from build123d import *

# Parameters (mm, degrees)
SKETCH1_W           = 59.0272
SKETCH1_H           = 30
BOSS_EXTRUDE1_DEPTH = 10
SKETCH2_R           = 2.1
CUT_EXTRUDE1_DEPTH  = 35.58399319
SKETCH3_R           = 1.7
CUT_EXTRUDE2_DEPTH  = 12
SKETCH4_R           = 1.65
CUT_EXTRUDE3_DEPTH  = 12
CUT_EXTRUDE4_DEPTH  = 2.5
CUT_EXTRUDE5_DEPTH  = 2.3
SKETCH7_R           = 3.5
CUT_EXTRUDE6_DEPTH  = 35.58399319
FILLET1_R           = 1
SKETCH8_W           = 39.5136
SKETCH8_H           = 30
CUT_EXTRUDE7_DEPTH  = 35.58399319


with BuildPart() as part:
    # Sketch1 → Boss-Extrude1 (new body)
    with BuildSketch(Plane(origin=(0, 0, 0), x_dir=(1, 0, 0), z_dir=(0, 1, 0))):
        Rectangle(SKETCH1_W, SKETCH1_H)
    extrude(amount=BOSS_EXTRUDE1_DEPTH)

    # Sketch2 → Cut-Extrude1 (cut, through all)
    with BuildSketch(Plane(origin=(0, 10, 0), x_dir=(1, 0, 0), z_dir=(0, 1, 0))):
        with Locations(Location((-6, -7.5, 0), (0, 0, 270))):
            Circle(SKETCH2_R)
        with Locations(Location((14, -7.5, 0), (0, 0, 270))):
            Circle(SKETCH2_R)
    extrude(amount=-CUT_EXTRUDE1_DEPTH, mode=Mode.SUBTRACT)

    # Sketch3 → Cut-Extrude2 (cut)
    with BuildSketch(Plane(origin=(29.5136, 0, 0), x_dir=(0, 0, -1), z_dir=(1, 0, 0))):
        with Locations((-10, 5)):
            Circle(SKETCH3_R)
        with Locations((10, 5)):
            Circle(SKETCH3_R)
    extrude(amount=-CUT_EXTRUDE2_DEPTH, mode=Mode.SUBTRACT)

    # Sketch4 → Cut-Extrude3 (cut)
    with BuildSketch(Plane.ZY.offset(29.5136)):
        with Locations((-10, 5)):
            Circle(SKETCH4_R)
        with Locations((10, 5)):
            Circle(SKETCH4_R)
    extrude(amount=-CUT_EXTRUDE3_DEPTH, mode=Mode.SUBTRACT)

    # Sketch5 → Cut-Extrude4 (cut)
    with BuildSketch(Plane(origin=(23.5136, 0, 0), x_dir=(0, 0, -1), z_dir=(1, 0, 0))):
        Polygon((-12.95, 6.703183294), (-12.95, 10), (-7.05, 10), (-7.05, 6.703183294), (-7.05, 3.296816706), (-10, 1.593633412), (-12.95, 3.296816706), align=None)
        Polygon((7.05, 6.703183294), (7.05, 3.296816706), (10, 1.593633412), (12.95, 3.296816706), (12.95, 6.703183294), (12.95, 10), (7.05, 10), align=None)
    extrude(amount=-CUT_EXTRUDE4_DEPTH, mode=Mode.SUBTRACT)

    # Sketch6 → Cut-Extrude5 (cut)
    with BuildSketch(Plane.ZY.offset(23.5136)):
        Polygon((-12.85, 6.645448267), (-12.85, 10), (-7.15, 10), (-7.15, 6.645448267), (-7.15, 3.354551733), (-10, 1.709103466), (-12.85, 3.354551733), align=None)
        Polygon((7.15, 6.645448267), (7.15, 3.354551733), (10, 1.709103466), (12.85, 3.354551733), (12.85, 6.645448267), (12.85, 10), (7.15, 10), align=None)
    extrude(amount=-CUT_EXTRUDE5_DEPTH, mode=Mode.SUBTRACT)

    # Sketch7 → Cut-Extrude6 (cut, through all)
    with BuildSketch(Plane(origin=(0, 10, 0), x_dir=(1, 0, 0), z_dir=(0, 1, 0))):
        with Locations(Location((9.7, 1.2, 0), (0, 0, 270))):
            Circle(SKETCH7_R)
        with Locations(Location((-15.7, 1.2, 0), (0, 0, 270))):
            Circle(SKETCH7_R)
    extrude(amount=-CUT_EXTRUDE6_DEPTH, mode=Mode.SUBTRACT)

    # Fillet1
    fillet1_edges = [part.edges().sort_by_distance(p)[0] for p in [
        (29.5136, 5, 15),
        (-29.5136, 5, 15),
        (-29.5136, 5, -15),
        (29.5136, 5, -15),
    ]]
    fillet(fillet1_edges, radius=FILLET1_R)

    # Sketch8 → Cut-Extrude7 (cut, through all)
    with BuildSketch(Plane(origin=(0, 10, 0), x_dir=(1, 0, 0), z_dir=(0, 1, 0))):
        with Locations((-9.7568, 0)):
            Rectangle(SKETCH8_W, SKETCH8_H)
    extrude(amount=-CUT_EXTRUDE7_DEPTH, mode=Mode.SUBTRACT)


solid = part.part
Check sheet for the modelled part. Datum: model origin and axes. Units: mm. A direction names the side the tool comes from. Round coordinates to 2 decimals unless told otherwise and drop trailing zeros. Loops run counter-clockwise (first coordinate to the right, second up) from the corner with the lowest first, then second, coordinate; pieces in that order, holes last. Notation, with made-up numbers: (0.25, -5.5) - (30.25, -5.5) arc R14 ccw to (30.25, 14.5) - close; hole circle Ø9 at (-20.5, 57). An arc over 180 degrees is marked (long way). Answer as CSV lines item,"result". Start each with the question number.
Item 1: Section check C-C (z = 7.5). Record the boundary of the cut face in (x, y), and give its area (3 significant figures).
Item 2: Scan lines: line 1 (X direction, y = 6.75, z = 7.5); line 2 (Z direction, x = 21.25, y = 4); line 3 (X direction, y = 8.75, z = -9.5). Record each from-to range of solid material in increasing order. Write a range as [from, to].
Item 3: Section check B-B (y = 1). Record the boundary of the cut face in (x, z), and give its area (3 significant figures).
Item 4: Section check A-A (x = 14). Record the boundary of the cut face in (y, z), and give its area (3 significant figures).
Item 5: Release check for a two-part mould opening along Y. For faces 1 (the flat face through (22.28, 2.43, 11.45)), 2 (the cylindrical face through (29.213, 5.07, -14.715)), 3 (the cylindrical face through (26.56, 3.34, -9.63)) record: +Y half, -Y half, draft (parallel to the pull), parting line (faces both ways), or undercut.
Item 6: Depth check by flat-ended pin: P1, Ø4, axis at y = 5, z = -10, coming from the +X side; P2, Ø2.5, axis at y = 5, z = 10, coming from the +X side. Enter the tip coordinate at first touch or a pass-through.
Item 7: Set-up check for faces 4 (the cylindrical face through (26.6, 3.5, 9.2)), 5 (the flat face through (22, 7, -7.05)), 6 (the flat face through (20, 10, 0)): record each of +Z, -Z, +X, -X, +Y, -Y from which the full face is reachable in a straight line by a thin tool's end or side.
Item 8: Section check D-D (x = 26). Record the boundary of the cut face in (y, z).
Report:
1,outline,"(10, 0) - (11.9, 0) - (11.9, 10) - (10, 10) - close; (16.1, 0) - (29.51, 0) - (29.51, 10) - (23.51, 10) - (23.51, 3.04) - (21.01, 3.04) - (21.01, 10) - (16.1, 10) - close"
1,area,"136 mm2"
2,line 1,"x = [10, 11.9], [16.1, 21.01], [23.51, 29.51]"
2,line 2,"z = [-15, -12.95], [-7.05, 7.05], [12.95, 15]"
2,line 3,"x = [10, 21.01], [23.51, 29.51]"
3,outline,"(10, -15) - (28.51, -15) arc R1 ccw to (29.51, -14) - (29.51, 14) arc R1 ccw to (28.51, 15) - (10, 15) - (10, 2.29) arc R3.5 cw to (10, -4.69) - close; hole circle Ø4.2 at (14, 7.5)"
3,area,"554 mm2"
4,outline,"(0, -15) - (10, -15) - (10, 5.4) - (0, 5.4) - close; (0, 9.6) - (10, 9.6) - (10, 15) - (0, 15) - close"
4,area,"258 mm2"
5,face 1,"+Y half"
5,face 2,"draft"
5,face 3,"undercut"
6,P1,"stops at x = 29.51"
6,P2,"stops at x = 17.51"
7,face 4,"+X"
7,face 5,"+Y"
7,face 6,"+Z, -Z, +X, -X, +Y"
8,outline,"(0, -15) - (10, -15) - (10, 15) - (0, 15) - close; hole circle Ø3.4 at (5, -10); hole circle Ø3.4 at (5, 10)"
